Read the model definition and answer for the solid it produces. Units are mm, in the model's axes. Face numbers are marked on the shaded views. A direction names the side the tool comes from. Round coordinates to 2 decimals unless told otherwise and drop trailing zeros. Write each loop counter-clockwise with the first axis right and the second up, starting at its lowest first coordinate (ties: lowest second). Pieces come first, ordered by that corner, then holes. Notation, with made-up numbers: (-28, -29) -> (7, -29) arc R27 ccw to (7, 6) -> close; hole circle Ø2 at (43, 9.5). An arc over 180 degrees is marked (long way). Return JSON: item names as keys, results as strings.
from build123d import *

# Parameters (mm, degrees)
BOSS_EXTRUDE1_DEPTH = 10
SKETCH2_R           = 3
BOSS_EXTRUDE2_DEPTH = 10


with BuildPart() as part:
    # Sketch1 → Boss-Extrude1 (new body)
    with BuildSketch(Plane(origin=(0, 0, 0), x_dir=(0, 0, -1), z_dir=(1, 0, 0))):
        with BuildLine():
            Line((-26, 0), (26, 0))
            Line((26, 0), (26, 32))
            ThreePointArc((26, 32), (23.656854249, 37.656854249), (18, 40))
            Line((18, 40), (-18, 40))
            ThreePointArc((-18, 40), (-23.656854249, 37.656854249), (-26, 32))
            Line((-26, 32), (-26, 0))
        make_face()
        with BuildLine():
            Line((-15, 32), (-15, 24))
            ThreePointArc((-15, 24), (-18, 21), (-21, 24))
            Line((-21, 24), (-21, 32))
            ThreePointArc((-21, 32), (-18, 35), (-15, 32))
        make_face(mode=Mode.SUBTRACT)
        with BuildLine():
            Line((15, 32), (15, 24))
            ThreePointArc((15, 24), (18, 21), (21, 24))
            Line((21, 24), (21, 32))
            ThreePointArc((21, 32), (18, 35), (15, 32))
        make_face(mode=Mode.SUBTRACT)
    extrude(amount=BOSS_EXTRUDE1_DEPTH)

    # Sketch2 → Boss-Extrude2 (add)
    with BuildSketch(Plane(origin=(0, 0, 0), x_dir=(1, 0, 0), z_dir=(0, 1, 0))):
        with BuildLine():
            Line((0, 26), (32, 26))
            ThreePointArc((32, 26), (35.514718626, 17.514718626), (44, 14))
            Line((44, 14), (88, 14))
            ThreePointArc((88, 14), (102, 0), (88, -14))
            Line((88, -14), (44, -14))
            ThreePointArc((44, -14), (35.514718626, -17.514718626), (32, -26))
            Line((32, -26), (0, -26))
            Line((0, -26), (0, 26))
        make_face()
        with Locations((20, 14)):
            Circle(SKETCH2_R, mode=Mode.SUBTRACT)
        with Locations((20, -14)):
            Circle(SKETCH2_R, mode=Mode.SUBTRACT)
        with BuildLine():
            Line((44, 6), (88, 6))
            ThreePointArc((88, 6), (94, 0), (88, -6))
            Line((88, -6), (44, -6))
            ThreePointArc((44, -6), (38, 0), (44, 6))
        make_face(mode=Mode.SUBTRACT)
    extrude(amount=BOSS_EXTRUDE2_DEPTH)


solid = part.part
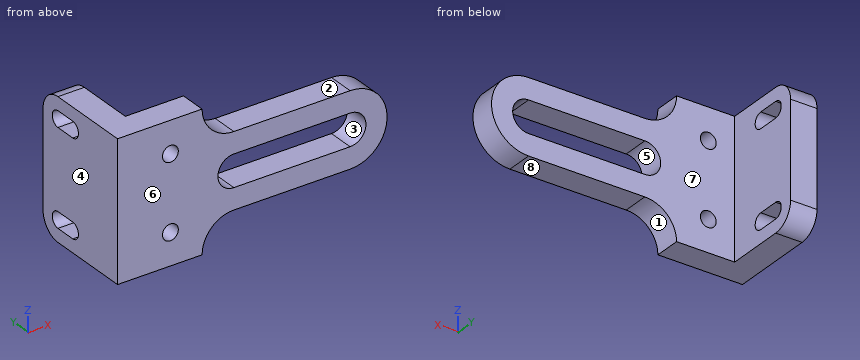
Item 1: Section A-A (y = 28.5) is taken. Give the vertices of the cut face in (x, z).
Worked answers:
{"outline": "(0, -26) -> (10, -26) -> (10, -21) -> (0, -21) -> close; (0, -15) -> (10, -15) -> (10, 15) -> (0, 15) -> close; (0, 21) -> (10, 21) -> (10, 26) -> (0, 26) -> close"}
Item 2: Straight lines are drawn through the part: L1, parallel to Z at x = 20, y = 8; L2, parallel to Z at x = 44, y = 3; L3, parallel to Y at x = 30.5, z = -1. For each, find the intervals that lie inside material, in ascending order. Write a range as [from, to].
Worked answers:
{"L1": "z = [-26, -17], [-11, 11], [17, 26]", "L2": "z = [-14, -6], [6, 14]", "L3": "y = [0, 10]"}
Item 3: A tool of negligible diameter and unlimited length cuts with its end or side. For the marked faces 4, 5, 6, 7 and 8, from which of +Z, -Z, +X, -X, +Y, -Y can it reach the whole face along a straight path? Write none if from no direction.
Worked answers:
{"face 4": "+Z, -Z, -X, +Y, -Y", "face 5": "+Y, -Y", "face 6": "+Z, -Z, +X, -X, -Y", "face 7": "+Z, -Z, +X, +Y", "face 8": "-Z, +X, +Y, -Y"}
Item 4: Flat-ended cylindrical pins translate along their axes: pin 1 (6 mm diameter, centred on y = 24.5, z = -14.5, fed in from +X); pin 2 (3 mm diameter, centred on x = 24, y = 12.5, fed in from +Z); pin 3 (3 mm diameter, centred on x = 72.5, y = 5.5, fed in from -Z); pin 4 (11 mm diameter, centred on x = 64.5, y = 4, fed in from +Z). Find the tip coordinate at first contact, or state that the pin passes through.
Worked answers:
{"pin 1": "stops at x = 10", "pin 2": "passes through", "pin 3": "stops at z = -14", "pin 4": "stops at z = 14"}
Item 5: Section C-C (y = 3) is taken. Give the vertices of the cut face in (x, z), then the cut area to 3 significant figures.
Worked answers:
{"outline": "(0, -26) -> (32, -26) arc R12 cw to (44, -14) -> (88, -14) arc R14 ccw to (88, 14) -> (44, 14) arc R12 cw to (32, 26) -> (0, 26) -> close; hole circle Ø6 at (20, -14); hole circle Ø6 at (20, 14); hole (44, -6) -> (88, -6) arc R6 ccw to (88, 6) -> (44, 6) arc R6 ccw to start", "area": "2,900 mm2"}
Item 6: Section B-B (x = 20) is taken. Give the vertices of the cut face in (y, z), then the cut area to 3 significant figures.
Worked answers:
{"outline": "(0, -26) -> (10, -26) -> (10, -17) -> (0, -17) -> close; (0, -11) -> (10, -11) -> (10, 11) -> (0, 11) -> close; (0, 17) -> (10, 17) -> (10, 26) -> (0, 26) -> close", "area": "400 mm2"}
Item 7: Section D-D (z = 12) is taken. Give the vertices of the cut face in (x, y), then the cut area to 3 significant figures.
Worked answers:
{"outline": "(0, 0) -> (17.76, 0) -> (17.76, 10) -> (10, 10) -> (10, 40) -> (0, 40) -> close; (22.24, 0) -> (95.21, 0) -> (95.21, 10) -> (22.24, 10) -> close", "area": "1,210 mm2"}
Item 8: For a pull along Z with two mould halves and no side action, classify the marked faces 1, 2 and 3 as released by +Z, released by -Z, zero draft, split by the parting line, or undercut.
Worked answers:
{"face 1": "released by -Z", "face 2": "released by +Z", "face 3": "undercut"}
